```python
from build123d import *

# Parameters (mm, degrees)
RESSALTO_EXTRUS_O1_DEPTH = 10
ESBO_O2_W                = 26.639233333
ESBO_O2_H                = 10
RESSALTO_EXTRUS_O2_DEPTH = 15
ESBO_O3_W                = 10
ESBO_O3_H                = 15
RESSALTO_EXTRUS_O3_DEPTH = 30
ESBO_O4_R                = 4.25
CORTE_EXTRUS_O1_DEPTH    = 30
FILETE1_R                = 5


with BuildPart() as part:
    # Esboço1 → Ressalto-extrusão1 (new body)
    with BuildSketch(Plane.XY):
        with BuildLine():
            Line((-26.689233333, 0), (-26.689233333, 10))
            Line((-26.689233333, 10), (-0.05, 10))
            ThreePointArc((-0.05, 10), (-0.014644661, 9.985355339), (0, 9.95))
            Line((0, 9.95), (0, 0.05))
            ThreePointArc((0, 0.05), (-0.014644661, 0.014644661), (-0.05, 0))
            Line((-0.05, 0), (-26.689233333, 0))
        make_face()
    extrude(amount=RESSALTO_EXTRUS_O1_DEPTH)

    # Esboço2 → Ressalto-extrusão2 (add)
    with BuildSketch(Plane.XZ):
        with Locations((-13.369616667, 5)):
            Rectangle(ESBO_O2_W, ESBO_O2_H)
    extrude(amount=RESSALTO_EXTRUS_O2_DEPTH)

    # Esboço3 → Ressalto-extrusão3 (add)
    with BuildSketch(Plane(origin=(-0.05, 0, 0), x_dir=(0, 0, -1), z_dir=(1, 0, 0))):
        with Locations((-5, -7.5)):
            Rectangle(ESBO_O3_W, ESBO_O3_H)
    extrude(amount=RESSALTO_EXTRUS_O3_DEPTH)

    # Esboço4 → Corte-extrusão1 (cut)
    with BuildSketch(Plane(origin=(0, 0, 0), x_dir=(-1, 0, 0), z_dir=(0, 0, -1))):
        with Locations((-25.08, -8.473337784)):
            Circle(ESBO_O4_R)
        with Locations((18.92, -8.473337784)):
            Circle(ESBO_O4_R)
    extrude(amount=-CORTE_EXTRUS_O1_DEPTH, mode=Mode.SUBTRACT)

    # Filete1
    filete1_edges = [part.edges().sort_by_distance(p)[0] for p in [
        (-26.689233333, -15, 5),
        (29.95, 0, 5),
        (29.95, -15, 5),
    ]]
    fillet(filete1_edges, radius=FILETE1_R)


solid = part.part
```
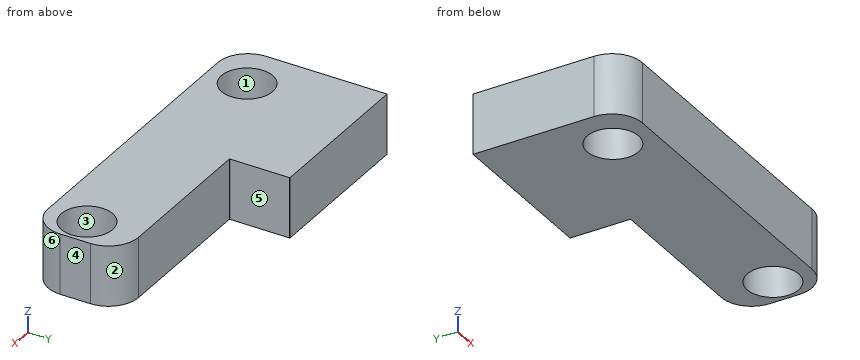
CAD build for the part. Positions are in the model's coordinates, mm. Face numbers are marked on the shaded views. A direction names the side the tool comes from. Round coordinates to 2 decimals unless told otherwise and drop trailing zeros. Loops run counter-clockwise (first coordinate to the right, second up) from the corner with the lowest first, then second, coordinate; pieces in that order, holes last. Notation, with made-up numbers: M 12.25,51 L 39.25,51 A14 cw 39.25,57 Z; hole C 88.25,-16 d5. An arc over 180 degrees is marked long. Return JSON: item names as keys, results as strings. Group by question number.
(1) Mould opens along Y. For the marked faces 1, 2, 3 and 4 say: +Y half, -Y half, draft (parallel to the pull), parting line (faces both ways), or undercut.
(2) Saw through at A-A, the plane x = -18.92. List the corners of the cut face in (y, z).
(3) Drop flat-ended pins along their axis: P1, Ø5, axis at x = 11, z = 6, coming from the +Y side; P2, Ø5, axis at y = 6, z = 5, coming from the +X side. Give the stop position or say it passes through.
(4) Wall check: probe 1 along X at (y, z) = (-8.25, 5.75); probe 2 along Y at (x, z) = (25.08, 4.5); probe 3 along X at (y, z) = (-7, 8). Give the ranges that are in metal, low to high. Write a range as [from, to].
(5) Saw through at B-B, the plane z = 1.75. List the corners of the cut face in (x, y).
(6) Tool access for the marked faces 5 and 6: list every direction of +Z, -Z, +X, -X, +Y, -Y with a clear straight run to the whole face (end or side of a thin tool).
(7) Saw through at C-C, the plane x = 8. List the corners of the cut face in (y, z).
Answer list:
{
 "1": {"face 1": "undercut", "face 2": "+Y half", "face 3": "undercut", "face 4": "draft"},
 "2": {"outline": "M -15,0 L -12.72,0 L -12.72,10 L -15,10 Z; M -4.22,0 L 10,0 L 10,10 L -4.22,10 Z"},
 "3": {"P1": "y = 0", "P2": "x = 0"},
 "4": {"probe 1": "[-26.69, -23.16], [-14.68, 20.84], [29.32, 29.95]", "probe 2": "[-15, -12.72], [-4.22, 0]", "probe 3": "[-26.69, -22.91], [-14.93, 21.09], [29.07, 29.95]"},
 "5": {"outline": "M -26.69,-10 A5 ccw -21.69,-15 L 24.95,-15 A5 ccw 29.95,-10 L 29.95,-5 A5 ccw 24.95,0 L -0.05,0 A0.05 ccw 0,0.05 L 0,9.95 A0.05 ccw -0.05,10 L -26.69,10 Z; hole C -18.92,-8.47 d8.5; hole C 25.08,-8.47 d8.5"},
 "6": {"face 5": "+Z, -Z, +X, +Y", "face 6": "+Z, -Z, +X, -Y"},
 "7": {"outline": "M -15,0 L 0,0 L 0,10 L -15,10 Z"}
}
